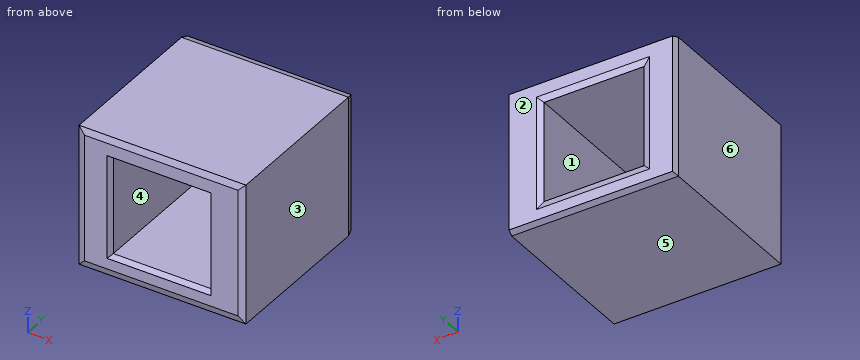
```python
from build123d import *
from OCP.BRepFilletAPI import BRepFilletAPI_MakeChamfer

# Parameters (mm, degrees)
SKETCH1_W           = 127
SKETCH1_H           = 106.690831556
BOSS_EXTRUDE1_DEPTH = 127
SKETCH3_W           = 76.2
SKETCH3_H           = 76.2
CUT_EXTRUDE1_DEPTH  = 165.203782008
CHAMFER1_SIZE       = 5.08
CHAMFER1_SIZE2      = 1.361181898


with BuildPart() as part:
    # Sketch1 → Boss-Extrude1 (new body)
    with BuildSketch(Plane(origin=(0, 0, 0), x_dir=(1, 0, 0), z_dir=(0, 1, 0))):
        with Locations((5.280383795, -24.777185501)):
            Rectangle(SKETCH1_W, SKETCH1_H)
    extrude(amount=BOSS_EXTRUDE1_DEPTH)

    # Sketch3 → Cut-Extrude1 (cut, through all)
    with BuildSketch(Plane(origin=(0, 0, 0), x_dir=(1, 0, 0), z_dir=(0, 1, 0))):
        with Locations((3.524009173, -24.106880488)):
            Rectangle(SKETCH3_W, SKETCH3_H)
    extrude(amount=CUT_EXTRUDE1_DEPTH, mode=Mode.SUBTRACT)

    # Chamfer1: one chamfer whose edges measure the first distance from different faces: ONE call of the kernel's chamfer builder (chamfer() names one face for all edges)
    chamfer1_edges_1 = [part.edges().sort_by_distance(p)[0] for p in [
        (68.780383795, 127, 24.777185501),
    ]]
    chamfer1_side_1 = [part.faces().sort_by_distance(p)[0] for p in [
        (68.780383795, 63.5, 24.777185501),
    ]]
    chamfer1_edges_2 = [part.edges().sort_by_distance(p)[0] for p in [
        (5.280383795, 127, -28.568230277),
    ]]
    chamfer1_side_2 = [part.faces().sort_by_distance(p)[0] for p in [
        (5.280383795, 63.5, -28.568230277),
    ]]
    chamfer1_edges_3 = [part.edges().sort_by_distance(p)[0] for p in [
        (41.624009173, 0, 24.106880488),
    ]]
    chamfer1_side_3 = [part.faces().sort_by_distance(p)[0] for p in [
        (41.624009173, 63.5, 24.106880488),
    ]]
    chamfer1_edges_4 = [part.edges().sort_by_distance(p)[0] for p in [
        (3.524009173, 0, -13.993119512),
    ]]
    chamfer1_side_4 = [part.faces().sort_by_distance(p)[0] for p in [
        (3.524009173, 63.5, -13.993119512),
    ]]
    chamfer1_edges_5 = [part.edges().sort_by_distance(p)[0] for p in [
        (-34.575990827, 0, 24.106880488),
    ]]
    chamfer1_side_5 = [part.faces().sort_by_distance(p)[0] for p in [
        (-34.575990827, 63.5, 24.106880488),
    ]]
    chamfer1_edges_6 = [part.edges().sort_by_distance(p)[0] for p in [
        (3.524009173, 0, 62.206880488),
    ]]
    chamfer1_side_6 = [part.faces().sort_by_distance(p)[0] for p in [
        (3.524009173, 63.5, 62.206880488),
    ]]
    chamfer1_edges_7 = [part.edges().sort_by_distance(p)[0] for p in [
        (41.624009173, 127, 24.106880488),
        (3.524009173, 127, -13.993119512),
        (-34.575990827, 127, 24.106880488),
        (3.524009173, 127, 62.206880488),
    ]]
    chamfer1_side_7 = [part.faces().sort_by_distance(p)[0] for p in [
        (5.280383795, 127, -26.909558111),
    ]]
    chamfer1_edges_8 = [part.edges().sort_by_distance(p)[0] for p in [
        (-58.219616205, 127, 24.777185501),
    ]]
    chamfer1_side_8 = [part.faces().sort_by_distance(p)[0] for p in [
        (-58.219616205, 63.5, 24.777185501),
    ]]
    chamfer1_edges_9 = [part.edges().sort_by_distance(p)[0] for p in [
        (5.280383795, 0, -28.568230277),
        (68.780383795, 0, 24.777185501),
        (5.280383795, 0, 78.122601279),
        (-58.219616205, 0, 24.777185501),
    ]]
    chamfer1_side_9 = [part.faces().sort_by_distance(p)[0] for p in [
        (5.280383795, 0, -26.909558111),
    ]]
    chamfer1_edges_10 = [part.edges().sort_by_distance(p)[0] for p in [
        (5.280383795, 127, 78.122601279),
    ]]
    chamfer1_side_10 = [part.faces().sort_by_distance(p)[0] for p in [
        (5.280383795, 63.5, 78.122601279),
    ]]
    chamfer1 = BRepFilletAPI_MakeChamfer(part.part.solid().wrapped)
    for e in chamfer1_edges_1:
        chamfer1.Add(CHAMFER1_SIZE, CHAMFER1_SIZE2, e.wrapped, chamfer1_side_1[0].wrapped)  # the first distance lies on this face
    for e in chamfer1_edges_2:
        chamfer1.Add(CHAMFER1_SIZE, CHAMFER1_SIZE2, e.wrapped, chamfer1_side_2[0].wrapped)  # the first distance lies on this face
    for e in chamfer1_edges_3:
        chamfer1.Add(CHAMFER1_SIZE, CHAMFER1_SIZE2, e.wrapped, chamfer1_side_3[0].wrapped)  # the first distance lies on this face
    for e in chamfer1_edges_4:
        chamfer1.Add(CHAMFER1_SIZE, CHAMFER1_SIZE2, e.wrapped, chamfer1_side_4[0].wrapped)  # the first distance lies on this face
    for e in chamfer1_edges_5:
        chamfer1.Add(CHAMFER1_SIZE, CHAMFER1_SIZE2, e.wrapped, chamfer1_side_5[0].wrapped)  # the first distance lies on this face
    for e in chamfer1_edges_6:
        chamfer1.Add(CHAMFER1_SIZE, CHAMFER1_SIZE2, e.wrapped, chamfer1_side_6[0].wrapped)  # the first distance lies on this face
    for e in chamfer1_edges_7:
        chamfer1.Add(CHAMFER1_SIZE, CHAMFER1_SIZE2, e.wrapped, chamfer1_side_7[0].wrapped)  # the first distance lies on this face
    for e in chamfer1_edges_8:
        chamfer1.Add(CHAMFER1_SIZE, CHAMFER1_SIZE2, e.wrapped, chamfer1_side_8[0].wrapped)  # the first distance lies on this face
    for e in chamfer1_edges_9:
        chamfer1.Add(CHAMFER1_SIZE, CHAMFER1_SIZE2, e.wrapped, chamfer1_side_9[0].wrapped)  # the first distance lies on this face
    for e in chamfer1_edges_10:
        chamfer1.Add(CHAMFER1_SIZE, CHAMFER1_SIZE2, e.wrapped, chamfer1_side_10[0].wrapped)  # the first distance lies on this face
    add(Compound.cast(chamfer1.Shape()), mode=Mode.REPLACE)


solid = part.part
```
Source: CAD feature listing. Evaluate the final solid. Frame: model axes, mm. Face numbers are marked on the shaded views. A direction names the side the tool comes from. Round coordinates to 2 decimals unless told otherwise and drop trailing zeros. Order: outer loops, then holes, each group sorted by start corner. A loop starts at its lowest first (then second) coordinate and runs counter-clockwise, first axis right, second up. Notation, with made-up numbers: (82.5, 68) -> (92.5, 68) arc R16 ccw to (92.5, 94) -> close; hole circle Ø8 at (-24.5, -26). An arc over 180 degrees is marked (long way). Use CSV: the item, a comma, the result in double quotes.
(1) Section B-B on x = -2.5. Return the cut outline in (y, z).
Report:
outline,"(0, -23.49) -> (1.36, -28.57) -> (121.92, -28.57) -> (127, -27.21) -> (127, -19.07) -> (125.64, -13.99) -> (5.08, -13.99) -> (0, -15.35) -> close; (0, 63.57) -> (5.08, 62.21) -> (125.64, 62.21) -> (127, 67.29) -> (127, 76.76) -> (121.92, 78.12) -> (1.36, 78.12) -> (0, 73.04) -> close"
(2) Ray query, L1, parallel to X at y = 75, z = 54; L2, parallel to Z at x = 12, y = 57; L3, parallel to Y at x = -39, z = 51.5. Return the intervals inside material, ascending.
Report:
L1,"-58.22 to -34.58, 41.62 to 68.78"
L2,"-28.57 to -13.99, 62.21 to 78.12"
L3,"0 to 126.82"
(3) Pull-direction query (X, two-part tool) for the marked faces 3, 4, 5 and 6; classes: +X half, -X half, draft (parallel to the pull), parting line (faces both ways), or undercut.
Report:
face 3,"+X half"
face 4,"undercut"
face 5,"draft"
face 6,"-X half"
(4) Access query for the marked faces 1 and 2. Directions: +Z, -Z, +X, -X, +Y, -Y. A direction counts if a zero-diameter tool reaches every point of the face in a straight line with its end or side. Return the directions, or none.
Report:
face 1,"+Y, -Y"
face 2,"+Z, -Z, +X, -X, +Y"
(5) Section A-A on y = 65. Return the cut outline in (x, z), and give its area (3 significant figures).
Report:
outline,"(-58.22, -28.57) -> (68.78, -28.57) -> (68.78, 78.12) -> (-58.22, 78.12) -> close; hole (-34.58, -13.99) -> (41.62, -13.99) -> (41.62, 62.21) -> (-34.58, 62.21) -> close"
area,"7,740 mm^2"
(6) Section C-C on z = 51. Return the cut outline in (x, y), and give its area (3 significant figures).
Report:
outline,"(-58.22, 1.36) -> (-53.14, 0) -> (-35.94, 0) -> (-34.58, 5.08) -> (-34.58, 125.64) -> (-39.66, 127) -> (-56.86, 127) -> (-58.22, 121.92) -> close; (41.62, 5.08) -> (42.99, 0) -> (63.7, 0) -> (68.78, 1.36) -> (68.78, 121.92) -> (67.42, 127) -> (46.7, 127) -> (41.62, 125.64) -> close"
area,"6,420 mm^2"
